from build123d import *

# Parameters (mm, degrees)
F0_W     = 12.7
F0_H     = 12.7
F1_DEPTH = 4.7625
F2_R     = 3.81
F3_R     = 1.25
F4_DEPTH = 58.421


with BuildPart() as f1:
    # F0 (on Top) → F1 (new body, symmetric)
    with BuildSketch(Plane.XY):
        Polygon((-48.768, 0), (0, 0), (0, -50.8), (3.81, -50.8), (3.81, -8.89), (3.81, 3.81), (-52.578, 3.81), (-52.578, -5.671398), (-48.768, -5.671398), align=None)
        Polygon((3.81, -50.8), (0, -50.8), (-3.81, -50.8), (0, -54.61), (3.81, -54.61), align=None)
        with Locations((10.16, -2.54)):
            Rectangle(F0_W, F0_H)
    extrude(amount=F1_DEPTH, both=True)

    # F2
    f2_edges = [f1.edges().sort_by_distance(p)[0] for p in [
        (16.51, -2.54, -4.7625),
        (16.51, -2.54, 4.7625),
    ]]
    fillet(f2_edges, radius=F2_R)

    # F3 (on face) → F4 (cut, through all)
    with BuildSketch(Plane(origin=(0, 3.81, 0), x_dir=(-1, 0, 0), z_dir=(0, 1, 0))):
        with Locations((-12.318778, 0)):
            Circle(F3_R)
    extrude(amount=-F4_DEPTH, mode=Mode.SUBTRACT)


solid = f1.part
Read the model definition and answer for the solid it produces. Units are mm, in the model's axes. A direction names the side the tool comes from. Round coordinates to 2 decimals unless told otherwise and drop trailing zeros. Order: outer loops, then holes, each group sorted by start corner. A loop starts at its lowest first (then second) coordinate and runs counter-clockwise, first axis right, second up.
1) Flat-ended cylindrical pins translate along their axes: pin 1 (3 mm diameter, centred on y = -24.5, z = -1.5, fed in from +X); pin 2 (3 mm diameter, centred on x = 12.32, z = 0, fed in from -Y); pin 3 (4 mm diameter, centred on x = -51, z = -1.5, fed in from -Y). Find the tip coordinate at first contact, or state that the pin passes through.
2) For faces 1 (the face through (-51, -5.671, 0)), 2 (the face through (10, -8.89, 0)), 3 (the face through (15.42, -2.45, 3.62)), determine the directions among +Z, -Z, +X, -X, +Y, -Y from which every point of the face is accessible in a straight line to the end or side of a thin tool.
3) The mould has two halves that part along Y. Classify faces 4 (the face through (-48.768, -3, 0)), 5 (the face through (-18, 3.81, 0)), 6 (the face through (-2, -50.8, 0)), 7 (the face through (0, -25, 0)): released by +Y, released by -Y, zero draft, split by the parting line, or undercut.
4) The part is cut by section A-A on z = 0. Write down the section's boundary in (x, y), plus the area to 3 significant figures.
5) The part is cut by section B-B on y = -23. Write down the section's boundary in (x, z).
6) Straight lines are drawn through the part: L1, parallel to X at y = -4.5, z = 0.25; L2, parallel to Y at x = -49, z = 4.25; L3, parallel to Y at x = -29, z = 0.5. For each, find the intervals that lie inside material, in ascending order.
Resolved:
1. pin 1: stops at x = 3.81
1. pin 2: stops at y = -8.89
1. pin 3: stops at y = -5.67
2. face 1: +Z, -Z, -X, -Y
2. face 2: +Z, -Z, +X, -Y
2. face 3: +Z, +X, +Y, -Y
3. face 4: zero draft
3. face 5: released by +Y
3. face 6: undercut
3. face 7: undercut
4. outline: (-52.58, -5.67) - (-48.77, -5.67) - (-48.77, 0) - (0, 0) - (0, -50.8) - (-3.81, -50.8) - (0, -54.61) - (3.81, -54.61) - (3.81, -8.89) - (11.07, -8.89) - (11.07, 3.81) - (-52.58, 3.81) - close; (13.57, -8.89) - (16.51, -8.89) - (16.51, 3.81) - (13.57, 3.81) - close
4. area: 581 mm2
5. outline: (0, -4.76) - (3.81, -4.76) - (3.81, 4.76) - (0, 4.76) - close
6. L1: x = -52.58 to -48.77, 0 to 11.09, 13.54 to 16.51
6. L2: y = -5.67 to 3.81
6. L3: y = 0 to 3.81
